Part model, mm, in its own coordinate system. A direction names the side the tool comes from. Round coordinates to 2 decimals unless told otherwise and drop trailing zeros. Order: outer loops, then holes, each group sorted by start corner. A loop starts at its lowest first (then second) coordinate and runs counter-clockwise, first axis right, second up. Notation, with made-up numbers: (40.5, 52) - (48.5, 52) arc R19 cw to (48.5, 81) - close; hole circle Ø10 at (76.25, 61). An arc over 180 degrees is marked (long way). Return JSON: item names as keys, results as strings. Group by question number.
Item 1: Tool access for faces 5 (the face through (100, 11, 1)), 6 (the face through (-97.93, 8.38, -69.35)), 7 (the face through (-1, 12, -65)): list every direction of +Z, -Z, +X, -X, +Y, -Y with a clear straight run to the whole face (end or side of a thin tool).
Item 2: Saw through at A-A on y = 11. List the corners of the cut face in (x, z), and give its area (3 significant figures).
Item 3: Drop flat-ended pins along their axis: pin 1 (5 mm diameter, centred on x = 20, z = 55, fed in from +Y); pin 2 (3.5 mm diameter, centred on x = 95, z = -70, fed in from -Y). Give the stop position or say it passes through.
Item 4: Saw through at B-B on x = 27. List the corners of the cut face in (y, z), and give its area (3 significant figures).
Item 5: Two-plate mould, pull along X, no slides. Class faces 1 (the face through (-1, 11, -75)), 2 (the face through (-1, 2, -1)), 3 (the face through (93.7, 17, 68.7)), 4 (the face through (-100, 11, 1)): released by +X, released by -X, zero draft, split by the parting line, or undercut.
Item 6: Probe probe 1 along X at (y, z) = (1.5, -45); probe 2 along Z at (x, y) = (66, 13); probe 3 along X at (y, z) = (10.5, -31.5). List the from-to ranges inside material, lowest first.
```python
from build123d import *

# Parameters (mm, degrees)
SKETCH1_W           = 200
SKETCH1_H           = 150
BOSS_EXTRUDE1_DEPTH = 2
SKETCH2_R           = 1.5
CUT_EXTRUDE1_DEPTH  = 126.015998976
SKETCH3_W           = 200
SKETCH3_H           = 150
SKETCH3_W_2         = 180
SKETCH3_H_2         = 130
BOSS_EXTRUDE2_DEPTH = 20
SKETCH4_R           = 1.5
CUT_EXTRUDE2_DEPTH  = 127.921235418
SKETCH5_R           = 3
CUT_EXTRUDE3_DEPTH  = 17


with BuildPart() as part:
    # Sketch1 → Boss-Extrude1 (new body)
    with BuildSketch(Plane(origin=(0, 0, 0), x_dir=(1, 0, 0), z_dir=(0, 1, 0))):
        Rectangle(SKETCH1_W, SKETCH1_H)
    extrude(amount=BOSS_EXTRUDE1_DEPTH)

    # Sketch2 → Cut-Extrude1 (cut, through all)
    with BuildSketch(Plane(origin=(0, 2, 0), x_dir=(1, 0, 0), z_dir=(0, 1, 0))):
        with Locations(Location((0, -5, 0), (0, 0, 270))):
            Circle(SKETCH2_R)
        with Locations(Location((0, -15, 0), (0, 0, 270))):
            Circle(SKETCH2_R)
        with Locations(Location((0, -25, 0), (0, 0, 270))):
            Circle(SKETCH2_R)
        with Locations(Location((0, -35, 0), (0, 0, 270))):
            Circle(SKETCH2_R)
        with Locations(Location((0, -45, 0), (0, 0, 270))):
            Circle(SKETCH2_R)
        with Locations(Location((0, -55, 0), (0, 0, 270))):
            Circle(SKETCH2_R)
        with Locations(Location((0, 55, 0), (0, 0, 90))):
            Circle(SKETCH2_R)
        with Locations(Location((0, 45, 0), (0, 0, 90))):
            Circle(SKETCH2_R)
        with Locations(Location((0, 35, 0), (0, 0, 90))):
            Circle(SKETCH2_R)
        with Locations(Location((0, 25, 0), (0, 0, 90))):
            Circle(SKETCH2_R)
        with Locations(Location((0, 15, 0), (0, 0, 90))):
            Circle(SKETCH2_R)
        with Locations(Location((0, 5, 0), (0, 0, 90))):
            Circle(SKETCH2_R)
        with Locations(Location((20, -55, 0), (0, 0, 90))):
            Circle(SKETCH2_R)
        with Locations(Location((20, -45, 0), (0, 0, 90))):
            Circle(SKETCH2_R)
        with Locations(Location((20, -35, 0), (0, 0, 90))):
            Circle(SKETCH2_R)
        with Locations(Location((20, -25, 0), (0, 0, 90))):
            Circle(SKETCH2_R)
        with Locations(Location((20, -15, 0), (0, 0, 90))):
            Circle(SKETCH2_R)
        with Locations(Location((20, -5, 0), (0, 0, 90))):
            Circle(SKETCH2_R)
        with Locations(Location((20, 5, 0), (0, 0, 270))):
            Circle(SKETCH2_R)
        with Locations(Location((20, 15, 0), (0, 0, 270))):
            Circle(SKETCH2_R)
        with Locations(Location((20, 25, 0), (0, 0, 270))):
            Circle(SKETCH2_R)
        with Locations(Location((20, 35, 0), (0, 0, 270))):
            Circle(SKETCH2_R)
        with Locations(Location((20, 45, 0), (0, 0, 270))):
            Circle(SKETCH2_R)
        with Locations(Location((20, 55, 0), (0, 0, 270))):
            Circle(SKETCH2_R)
        with Locations(Location((-20, -55, 0), (0, 0, 90))):
            Circle(SKETCH2_R)
        with Locations(Location((-20, -45, 0), (0, 0, 90))):
            Circle(SKETCH2_R)
        with Locations(Location((-20, -35, 0), (0, 0, 90))):
            Circle(SKETCH2_R)
        with Locations(Location((-20, -25, 0), (0, 0, 90))):
            Circle(SKETCH2_R)
        with Locations(Location((-20, -15, 0), (0, 0, 90))):
            Circle(SKETCH2_R)
        with Locations(Location((-20, -5, 0), (0, 0, 90))):
            Circle(SKETCH2_R)
        with Locations(Location((-20, 5, 0), (0, 0, 270))):
            Circle(SKETCH2_R)
        with Locations(Location((-20, 15, 0), (0, 0, 270))):
            Circle(SKETCH2_R)
        with Locations(Location((-20, 25, 0), (0, 0, 270))):
            Circle(SKETCH2_R)
        with Locations(Location((-20, 35, 0), (0, 0, 270))):
            Circle(SKETCH2_R)
        with Locations(Location((-20, 45, 0), (0, 0, 270))):
            Circle(SKETCH2_R)
        with Locations(Location((-20, 55, 0), (0, 0, 270))):
            Circle(SKETCH2_R)
        with Locations(Location((40, -35, 0), (0, 0, 270))):
            Circle(SKETCH2_R)
        with Locations(Location((40, -45, 0), (0, 0, 270))):
            Circle(SKETCH2_R)
        with Locations(Location((40, -55, 0), (0, 0, 270))):
            Circle(SKETCH2_R)
        with Locations(Location((40, -5, 0), (0, 0, 270))):
            Circle(SKETCH2_R)
        with Locations(Location((40, -15, 0), (0, 0, 270))):
            Circle(SKETCH2_R)
        with Locations(Location((40, -25, 0), (0, 0, 270))):
            Circle(SKETCH2_R)
        with Locations(Location((40, 25, 0), (0, 0, 90))):
            Circle(SKETCH2_R)
        with Locations(Location((40, 15, 0), (0, 0, 90))):
            Circle(SKETCH2_R)
        with Locations(Location((40, 5, 0), (0, 0, 90))):
            Circle(SKETCH2_R)
        with Locations(Location((40, 55, 0), (0, 0, 90))):
            Circle(SKETCH2_R)
        with Locations(Location((40, 45, 0), (0, 0, 90))):
            Circle(SKETCH2_R)
        with Locations(Location((40, 35, 0), (0, 0, 90))):
            Circle(SKETCH2_R)
        with Locations(Location((-40, -55, 0), (0, 0, 270))):
            Circle(SKETCH2_R)
        with Locations(Location((-40, -45, 0), (0, 0, 270))):
            Circle(SKETCH2_R)
        with Locations(Location((-40, -35, 0), (0, 0, 270))):
            Circle(SKETCH2_R)
        with Locations(Location((-40, -25, 0), (0, 0, 270))):
            Circle(SKETCH2_R)
        with Locations(Location((-40, -15, 0), (0, 0, 270))):
            Circle(SKETCH2_R)
        with Locations(Location((-40, -5, 0), (0, 0, 270))):
            Circle(SKETCH2_R)
        with Locations(Location((-40, 15, 0), (0, 0, 90))):
            Circle(SKETCH2_R)
        with Locations(Location((-40, 5, 0), (0, 0, 90))):
            Circle(SKETCH2_R)
        with Locations(Location((-40, 35, 0), (0, 0, 90))):
            Circle(SKETCH2_R)
        with Locations(Location((-40, 25, 0), (0, 0, 90))):
            Circle(SKETCH2_R)
        with Locations(Location((-40, 55, 0), (0, 0, 90))):
            Circle(SKETCH2_R)
        with Locations(Location((-40, 45, 0), (0, 0, 90))):
            Circle(SKETCH2_R)
    extrude(amount=-CUT_EXTRUDE1_DEPTH, mode=Mode.SUBTRACT)

    # Sketch3 → Boss-Extrude2 (add)
    with BuildSketch(Plane(origin=(0, 2, 0), x_dir=(1, 0, 0), z_dir=(0, 1, 0))):
        Rectangle(SKETCH3_W, SKETCH3_H)
        Rectangle(SKETCH3_W_2, SKETCH3_H_2, mode=Mode.SUBTRACT)
    extrude(amount=BOSS_EXTRUDE2_DEPTH)

    # Sketch4 → Cut-Extrude2 (cut, through all)
    with BuildSketch(Plane.XZ):
        with Locations(Location((95, 70, 0), (0, 0, 270))):
            Circle(SKETCH4_R)
        with Locations(Location((95, -70, 0), (0, 0, 270))):
            Circle(SKETCH4_R)
        with Locations(Location((-95, 70, 0), (0, 0, 270))):
            Circle(SKETCH4_R)
        with Locations(Location((-95, -70, 0), (0, 0, 270))):
            Circle(SKETCH4_R)
        with Locations(Location((95, 0, 0), (0, 0, 270))):
            Circle(SKETCH4_R)
        with Locations(Location((-95, 0, 0), (0, 0, 270))):
            Circle(SKETCH4_R)
    extrude(amount=-CUT_EXTRUDE2_DEPTH, mode=Mode.SUBTRACT)

    # Sketch5 → Cut-Extrude3 (cut)
    with BuildSketch(Plane.XZ):
        with Locations(Location((95, 70, 0), (0, 0, 270))):
            Circle(SKETCH5_R)
        with Locations(Location((95, -70, 0), (0, 0, 270))):
            Circle(SKETCH5_R)
        with Locations(Location((-95, 70, 0), (0, 0, 270))):
            Circle(SKETCH5_R)
        with Locations(Location((-95, -70, 0), (0, 0, 270))):
            Circle(SKETCH5_R)
    extrude(amount=-CUT_EXTRUDE3_DEPTH, mode=Mode.SUBTRACT)


solid = part.part
```
Filled in:
{
 "1": {"face 5": "+Z, -Z, +X, +Y, -Y", "face 6": "-Y", "face 7": "+Y"},
 "2": {"outline": "(-100, -75) - (100, -75) - (100, 75) - (-100, 75) - close; hole circle Ø6 at (-95, -70); hole circle Ø6 at (-95, 70); hole circle Ø3 at (-95, 0); hole (-90, -65) - (90, -65) - (90, 65) - (-90, 65) - close; hole circle Ø6 at (95, -70); hole circle Ø6 at (95, 70); hole circle Ø3 at (95, 0)", "area": "6,470 mm^2"},
 "3": {"pin 1": "stops at y = 2", "pin 2": "stops at y = 17"},
 "4": {"outline": "(0, -75) - (22, -75) - (22, -65) - (2, -65) - (2, 65) - (22, 65) - (22, 75) - (0, 75) - close", "area": "700 mm^2"},
 "5": {"face 1": "zero draft", "face 2": "undercut", "face 3": "undercut", "face 4": "released by -X"},
 "6": {"probe 1": "x = -100 to -41.5, -38.5 to -21.5, -18.5 to -1.5, 1.5 to 18.5, 21.5 to 38.5, 41.5 to 100", "probe 2": "z = -75 to -65, 65 to 75", "probe 3": "x = -100 to -90, 90 to 100"}
}
